from build123d import *

# Parameters (mm, degrees)
F0_W          = 50
F0_H          = 50
F1_DEPTH      = 900
F3_DEPTH      = 25.001
F3_DEPTH_BACK = 25.001
F5_DEPTH      = 25.001
F5_DEPTH_BACK = 25.001


with BuildPart() as f1:
    # F0 (on Top) → F1 (new body)
    with BuildSketch(Plane.XY):
        Rectangle(F0_W, F0_H)
    extrude(amount=F1_DEPTH)

    # F2 (on Right) → F3 (cut, two sides)
    with BuildSketch(Plane.YZ) as f3_sk:
        Polygon((135.3058686236, 900), (-25, 900), (135.3058686236, 739.6941313764), align=None)
    extrude(amount=-F3_DEPTH, mode=Mode.SUBTRACT)
    extrude(f3_sk.sketch, amount=F3_DEPTH_BACK, mode=Mode.SUBTRACT)

    # F4 (on Right) → F5 (cut, two sides)
    with BuildSketch(Plane.YZ) as f5_sk:
        Polygon((25, 50), (-25, 0), (25, 0), align=None)
    extrude(amount=-F5_DEPTH, mode=Mode.SUBTRACT)
    extrude(f5_sk.sketch, amount=F5_DEPTH_BACK, mode=Mode.SUBTRACT)


solid = f1.part
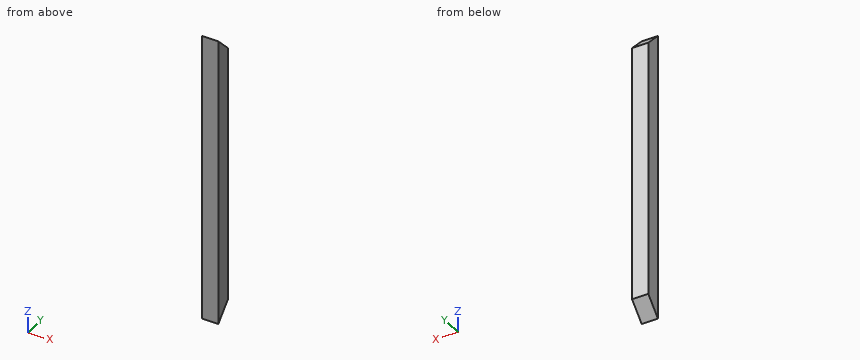
Part model, mm, in its own coordinate system. Give positions to 0.01 mm unless a question says otherwise; leave off trailing zeros. Order: outer loops, then holes, each group sorted by start corner. A loop starts at its lowest first (then second) coordinate and runs counter-clockwise, first axis right, second up. Notation, with made-up numbers: (43, 2.5) -> (57, 2.5) arc R25 cw to (57, 34.5) -> close; hole circle Ø2 at (-4.5, -32.75). An arc over 180 degrees is marked (long way). Use one line per item in the form item = value.
(1) Drill centre lines: line 1 (Z direction, x = 17, y = 15); line 2 (Z direction, x = -22, y = 21). Where is each one in solid material? Low to high. Write a range as from..to.
Solution:
line_1 = 40..860
line_2 = 46..854
(2) Saw through at B-B (x = 12). Write the cut outline in (y, z).
Solution:
outline = (-25, 0) -> (25, 50) -> (25, 850) -> (-25, 900) -> close
(3) Flat gauge pins, fed straight in: P1, Ø5, axis at x = -16.5, y = -15, coming from the +Z side; P2, Ø3, axis at x = -7.5, y = -5.5, coming from the +Z side; P3, Ø1.5, axis at x = -14.5, y = 3.5, coming from the +Z side. Where does each tip first touch, or does it go through?
Solution:
P1 = 892.5
P2 = 882
P3 = 872.25
(4) Saw through at A-A (y = -7). Write the cut outline in (x, z).
Solution:
outline = (-25, 18) -> (25, 18) -> (25, 882) -> (-25, 882) -> close
